Geometry check sheet. Reference: drawing and pictorial views, mm from the part's lowest x, y, z. A direction names the side the tool comes from. Round coordinates to 2 decimals unless told otherwise and drop trailing zeros. Write each loop counter-clockwise with the first axis right and the second up, starting at its lowest first coordinate (ties: lowest second). Pieces come first, ordered by that corner, then holes. Notation, with made-up numbers: (-1.5, -33.5) - (10.5, -33.5) arc R12 ccw to (10.5, -28.5) - close; hole circle Ø5 at (19, 7.25). An arc over 180 degrees is marked (long way). Return JSON: item names as keys, results as strings.
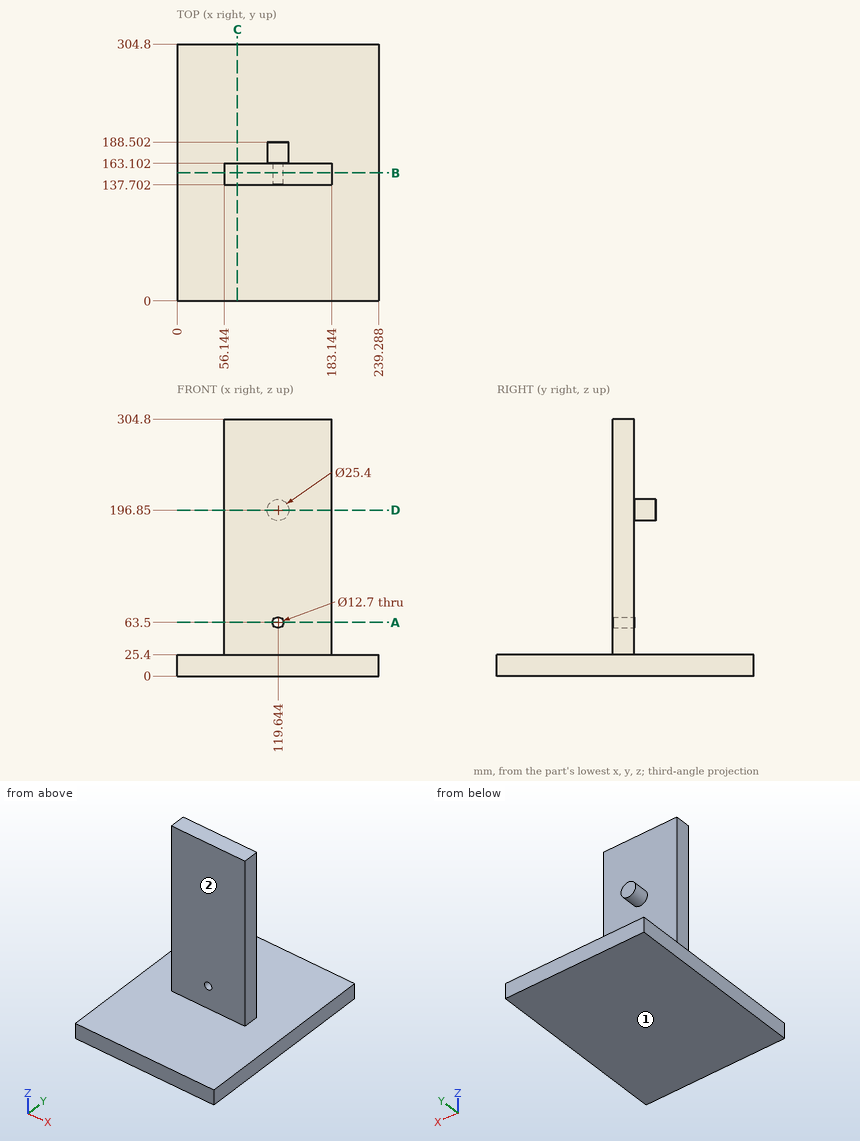
(1) Section check A-A, the plane z = 63.5. Enter the section's corners in (x, y), plus the area to 3 significant figures.
Response values:
{"outline": "(56.14, 137.7) - (113.29, 137.7) - (113.29, 163.1) - (56.14, 163.1) - close; (125.99, 137.7) - (183.14, 137.7) - (183.14, 163.1) - (125.99, 163.1) - close", "area": "2,900 mm^2"}
(2) Material ranges on line 1 along Z through (x, y) = (44.5, 121); line 2 along Y through (x, z) = (98, 108), recorded low to high. Write a range as [from, to].
Response values:
{"line 1": "z = [0, 25.4]", "line 2": "y = [137.7, 163.1]"}
(3) Access from +Z, -Z, +X, -X, +Y, -Y to the whole of each face (thin tool, end or side, straight path). Record for the marked faces 1 and 2.
Response values:
{"face 1": "-Z, +X, -X, +Y, -Y", "face 2": "+Z, +X, -X, -Y"}
(4) Section check C-C, the plane x = 71.5. Enter the section's corners in (y, z).
Response values:
{"outline": "(0, 0) - (304.8, 0) - (304.8, 25.4) - (163.1, 25.4) - (163.1, 304.8) - (137.7, 304.8) - (137.7, 25.4) - (0, 25.4) - close"}
(5) Gauge pin test, flat ends, axial feed: pin 1 (10 mm diameter, centred on x = 94.5, z = 45, fed in from -Y); pin 2 (8 mm diameter, centred on x = 56.5, z = 76.5, fed in from +Y); pin 3 (8 mm diameter, centred on y = 147, z = 235, fed in from +X). Record the tip position at first contact, or that the pin passes through.
Response values:
{"pin 1": "stops at y = 137.7", "pin 2": "stops at y = 163.1", "pin 3": "stops at x = 183.14"}
(6) Section check D-D, the plane z = 196.85. Enter the section's corners in (x, y).
Response values:
{"outline": "(56.14, 137.7) - (183.14, 137.7) - (183.14, 163.1) - (132.34, 163.1) - (132.34, 188.5) - (106.94, 188.5) - (106.94, 163.1) - (56.14, 163.1) - close"}
(7) Section check B-B, the plane y = 152. Enter the section's corners in (x, z).
Response values:
{"outline": "(0, 0) - (239.29, 0) - (239.29, 25.4) - (183.14, 25.4) - (183.14, 304.8) - (56.14, 304.8) - (56.14, 25.4) - (0, 25.4) - close; hole circle Ø12.7 at (119.64, 63.5)"}
